```python
from build123d import *

# Parameters (mm, degrees)
SKETCH1_R           = 2
BOSS_EXTRUDE1_DEPTH = 2
SKETCH2_R           = 1.5
BOSS_EXTRUDE2_DEPTH = 1.5
SKETCH3_R           = 1
BOSS_EXTRUDE3_DEPTH = 13
SKETCH4_R           = 0.125
BOSS_EXTRUDE4_DEPTH = 13


with BuildPart() as part:
    # Sketch1 → Boss-Extrude1 (new body)
    with BuildSketch(Plane(origin=(0, 0, 0), x_dir=(1, 0, 0), z_dir=(0, 1, 0))):
        Circle(SKETCH1_R)
    extrude(amount=BOSS_EXTRUDE1_DEPTH)

    # Sketch2 → Boss-Extrude2 (add)
    with BuildSketch(Plane(origin=(0, 2, 0), x_dir=(1, 0, 0), z_dir=(0, 1, 0))):
        Circle(SKETCH2_R)
    extrude(amount=BOSS_EXTRUDE2_DEPTH)

    # Sketch3 → Boss-Extrude3 (add)
    with BuildSketch(Plane(origin=(0, 3.5, 0), x_dir=(1, 0, 0), z_dir=(0, 1, 0))):
        Circle(SKETCH3_R)
    extrude(amount=BOSS_EXTRUDE3_DEPTH)

    # Sketch4 → Boss-Extrude4 (add)
    with BuildSketch(Plane(origin=(0, 16.5, 0), x_dir=(1, 0, 0), z_dir=(0, 1, 0))):
        with Locations((0, 1)):
            Circle(SKETCH4_R)
        with Locations((-1, 0)):
            Circle(SKETCH4_R)
        with Locations((0, -1)):
            Circle(SKETCH4_R)
        with Locations((1, 0)):
            Circle(SKETCH4_R)
    extrude(amount=-BOSS_EXTRUDE4_DEPTH)


solid = part.part
```
For this review, take the finished solid that the model builds, in its own axes (mm). A direction names the side the tool comes from. Round coordinates to 2 decimals unless told otherwise and drop trailing zeros. Write each loop counter-clockwise with the first axis right and the second up, starting at its lowest first coordinate (ties: lowest second). Pieces come first, ordered by that corner, then holes. Notation, with made-up numbers: (82, 34) - (96, 34) arc R28 ccw to (96, 69) - close; hole circle Ø6 at (71, 62). An arc over 180 degrees is marked (long way). Use CSV: the item, a comma, the result in double quotes.
1) Add section C-C on z = 0.8. Write out the cut boundary in (x, y), and give its area (3 significant figures).
Conclusion:
outline,"(-1.83, 0) - (1.83, 0) - (1.83, 2) - (1.27, 2) - (1.27, 3.5) - (0.6, 3.5) - (0.6, 16.5) - (-0.6, 16.5) - (-0.6, 3.5) - (-1.27, 3.5) - (-1.27, 2) - (-1.83, 2) - close"
area,"26.7 mm^2"
2) For faces 1 (the cylindrical face through (0.714, 9.909, -0.701)), 2 (the cylindrical face through (-0.714, 9.909, 0.701)), 3 (the flat face through (0.6, 3.5, 1)), list the 3-axis set-ups (+Z, -Z, +X, -X, +Y, -Y) from which the entire face can be reached by the end or side of a thin tool; tool diameter is ignored.
Conclusion:
face 1,"-Z, +X, +Y"
face 2,"+Z, -X, +Y"
face 3,"+Y"
3) Add section D-D on x = -1.3. Write out the cut boundary in (y, z).
Conclusion:
outline,"(0, -1.52) - (2, -1.52) - (2, -0.75) - (3.5, -0.75) - (3.5, 0.75) - (2, 0.75) - (2, 1.52) - (0, 1.52) - close"
4) Wall thickness on line 1 along Y through (x, z) = (-1.5, 0.45); line 2 along X through (y, z) = (7.75, 0.35); line 3 along X through (y, z) = (10.25, -0.9): over which ranges is each line inside the solid? List them lowest first. Write a range as from..to.
Conclusion:
line 1,"y = 0..2"
line 2,"x = -0.94..0.94"
line 3,"x = -0.44..0.44"
5) Add section A-A on y = 10.5. Write out the cut boundary in (x, z) (3 decimals), and give its area (3 significant figures).
Conclusion:
outline,"(-0.992, -0.125) arc R1 ccw to (-0.125, -0.992) arc R0.125 ccw (long way) to (0.125, -0.992) arc R1 ccw to (0.992, -0.125) arc R0.125 ccw (long way) to (0.992, 0.125) arc R1 ccw to (0.125, 0.992) arc R0.125 ccw (long way) to (-0.125, 0.992) arc R1 ccw to (-0.992, 0.125) arc R0.125 ccw (long way) to start"
area,"3.24 mm^2"
6) Add section B-B on x = 0.7. Write out the cut boundary in (y, z).
Conclusion:
outline,"(0, -1.87) - (2, -1.87) - (2, -1.33) - (3.5, -1.33) - (3.5, -0.71) - (16.5, -0.71) - (16.5, 0.71) - (3.5, 0.71) - (3.5, 1.33) - (2, 1.33) - (2, 1.87) - (0, 1.87) - close"
7) Clearance check with flat-ended pins moving along their axes: pin 1 Ø2 at (x, y) = (-0.5, 3.5) entering from +Z; pin 2 Ø2 at (y, z) = (8.5, 0) entering from -X (3 decimals). State where each tip first meets the part, or that it passes through.
Conclusion:
pin 1,"stops at z = 1.5"
pin 2,"stops at x = -1.125"
